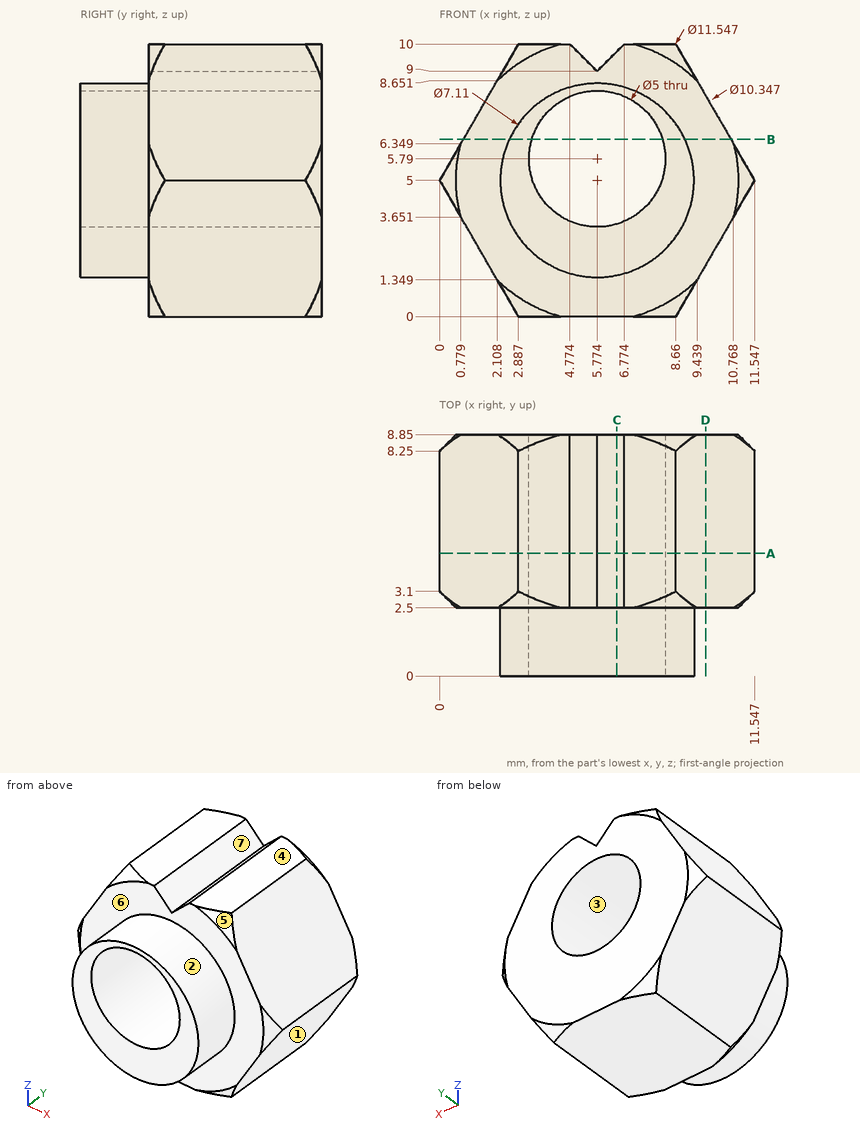
Verification items for this drawing (mm, ordinates from the low corner). A direction names the side the tool comes from. Coordinates: 2 decimals unless noted, no trailing zeros. Order: outer loops, then holes, each group sorted by start corner. A loop starts at its lowest first (then second) coordinate and runs counter-clockwise, first axis right, second up. Notation, with made-up numbers: (11.5, 67.5) - (24.5, 67.5) arc R18 ccw to (24.5, 97.5) - close; hole circle Ø4 at (-34.75, 9). An arc over 180 degrees is marked (long way). Answer in a Markdown table with one row per item. Add a question column.
1. Gauge pin test, flat ends, axial feed: pin 1 Ø5 at (y, z) = (3, 2) entering from +X; pin 2 Ø4 at (x, y) = (10, 1.5) entering from +Z; pin 3 Ø3 at (x, z) = (5.5, 5) entering from -Y. Record the tip position at first contact, or that the pin passes through.
2. Draft check along X on the marked faces 1, 2, 3 and 4. Enter one of: +X half, -X half, draft (parallel to the pull), parting line (faces both ways), or undercut.
3. Section check C-C (x = 6.5). Enter the section's corners in (y, z).
4. Section check A-A (y = 4.5). Enter the section's corners in (x, z).
5. Section check B-B (z = 6.5). Enter the section's corners in (x, y).
6. Material ranges on L1, parallel to Y at x = 3.5, z = 9.5; L2, parallel to X at y = 7.5, z = 9.75 (1 decimal); L3, parallel to Z at x = 5, y = 1, recorded low to high. Write a range as [from, to].
7. Access from +Z, -Z, +X, -X, +Y, -Y to the whole of each face (thin tool, end or side, straight path). Record for the marked faces 5, 6 and 7.
8. Section check D-D (x = 9.75). Enter the section's corners in (y, z).
Data:
| question | item | result |
|---|---|---|
| 1 | pin 1 | stops at x = 11.26 |
| 1 | pin 2 | stops at z = 9.89 |
| 1 | pin 3 | passes through |
| 2 | face 1 | +X half |
| 2 | face 2 | parting line |
| 2 | face 3 | undercut |
| 2 | face 4 | draft |
| 3 | outline | (0, 1.52) - (2.5, 1.52) - (2.5, 0) - (8.85, 0) - (8.85, 3.4) - (0, 3.4) - close; (0, 8.18) - (8.85, 8.18) - (8.85, 9.73) - (2.5, 9.73) - (2.5, 8.48) - (0, 8.48) - close |
| 4 | outline | (0, 5) - (2.89, 0) - (8.66, 0) - (11.55, 5) - (8.66, 10) - (6.77, 10) - (5.77, 9) - (4.77, 10) - (2.89, 10) - close; hole circle Ø5 at (5.77, 5.79) |
| 5 | outline | (0.87, 2.5) - (2.55, 2.5) - (2.55, 0) - (3.38, 0) - (3.38, 8.85) - (0.87, 8.85) - close; (8.17, 0) - (9, 0) - (9, 2.5) - (10.68, 2.5) - (10.68, 8.85) - (8.17, 8.85) - close |
| 6 | L1 | y = [2.5, 8.85] |
| 6 | L2 | x = [2.7, 5], [6.5, 8.8] |
| 6 | L3 | z = [1.53, 3.41], [8.17, 8.47] |
| 7 | face 5 | +Z, +X, -Y |
| 7 | face 6 | -Y |
| 7 | face 7 | +Z, +Y, -Y |
| 8 | outline | (2.5, 1.89) - (8.85, 1.89) - (8.85, 8.11) - (2.5, 8.11) - close |
